Print and shaded views of the part. All mm, measured from the part's lowest x, y and z. A direction names the side the tool comes from. Coordinates: 2 decimals unless noted, no trailing zeros. Order: outer loops, then holes, each group sorted by start corner. A loop starts at its lowest first (then second) coordinate and runs counter-clockwise, first axis right, second up. Notation, with made-up numbers: M -34,76.25 L -2,76.25 A10 ccw -2,81.25 Z; hole C 80,-3 d11. An arc over 180 degrees is marked long. One line per item, written item: value.
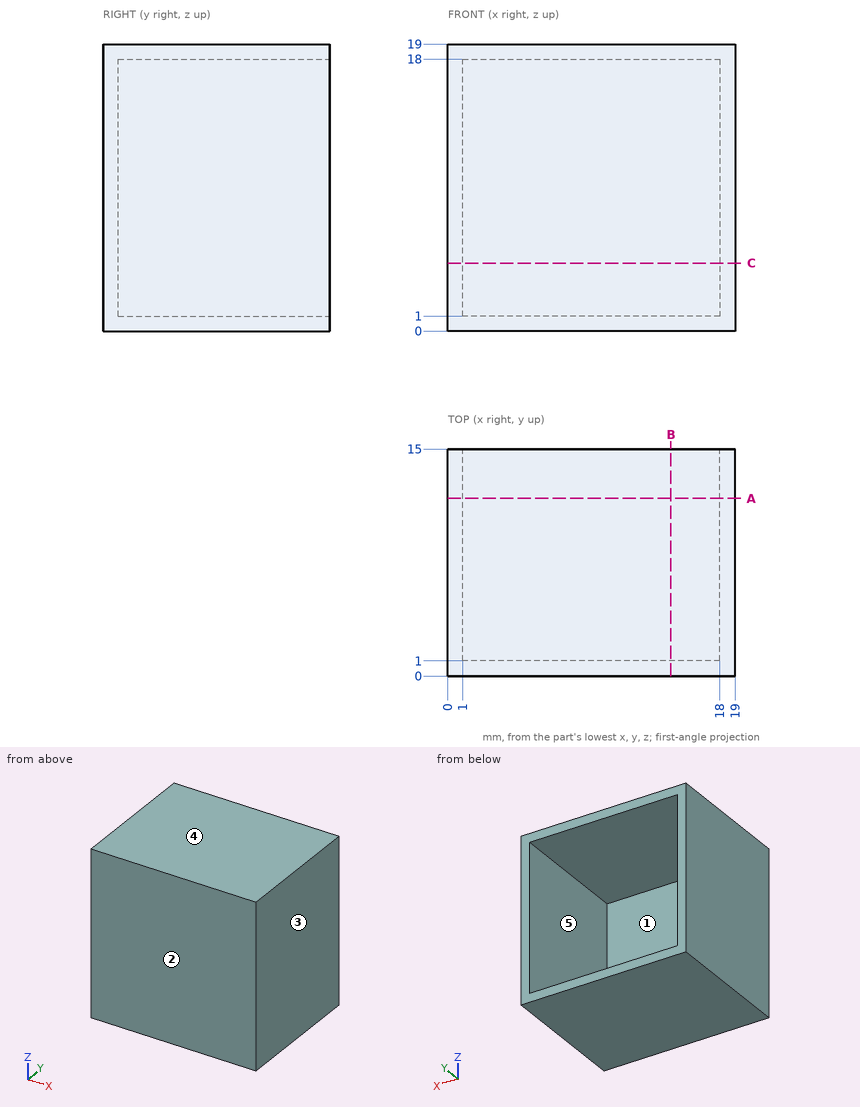
Q1. Mould opens along Z. For the marked faces 3, 4 and 5 say: released by +Z, released by -Z, zero draft, split by the parting line, or undercut.
Recorded:
face 3: zero draft
face 4: released by +Z
face 5: undercut
Q2. Slice it at A-A (y = 11.75). List the corners of the cut face in (x, z).
Recorded:
outline: M 0,0 L 19,0 L 19,19 L 0,19 Z; hole M 1,1 L 18,1 L 18,18 L 1,18 Z
Q3. Pin check, flat tips, straight feed: pin 1 Ø6 at (x, z) = (14.5, 16.5) entering from -Y; pin 2 Ø1.5 at (x, z) = (12, 16.5) entering from +Y. Stop position of each tip, or through.
Recorded:
pin 1: stops at y = 0
pin 2: stops at y = 1
Q4. Drill centre lines: line 1 along X through (y, z) = (4.75, 11.5); line 2 along Y through (x, z) = (16.75, 17). Where is each one in solid material? Low to high.
Recorded:
line 1: x = 0 to 1, 18 to 19
line 2: y = 0 to 1
Q5. Slice it at B-B (x = 14.75). List the corners of the cut face in (y, z), plus the area to 3 significant figures.
Recorded:
outline: M 0,0 L 15,0 L 15,1 L 1,1 L 1,18 L 15,18 L 15,19 L 0,19 Z
area: 47.0 mm^2
Q6. Slice it at C-C (z = 4.5). List the corners of the cut face in (x, y), plus the area to 3 significant figures.
Recorded:
outline: M 0,0 L 19,0 L 19,15 L 18,15 L 18,1 L 1,1 L 1,15 L 0,15 Z
area: 47.0 mm^2
Q7. Which spindle directions (+Z, -Z, +X, -X, +Y, -Y) get a long thin tool onto all of the face, cutting with end or side? Do the marked faces 1 and 2. Say none if no direction does.
Recorded:
face 1: +Y
face 2: +Z, -Z, +X, -X, -Y
